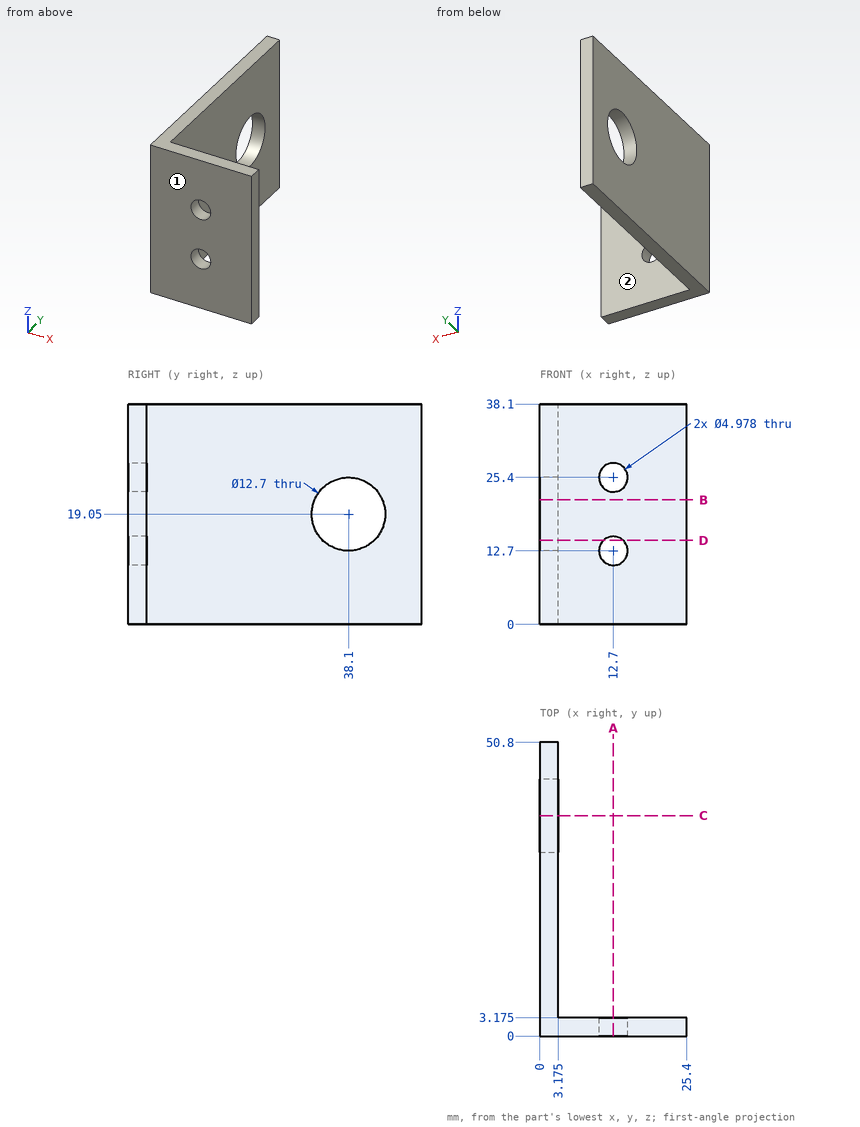
Part print with two shaded views. Sizes in mm from the minimum x, y, z corner. A direction names the side the tool comes from. Round coordinates to 2 decimals unless told otherwise and drop trailing zeros. Order: outer loops, then holes, each group sorted by start corner. A loop starts at its lowest first (then second) coordinate and runs counter-clockwise, first axis right, second up. Notation, with made-up numbers: M -11,-10.75 L 22,-10.75 A26 ccw 22,12.25 Z; hole C -27,-25.75 d3. An arc over 180 degrees is marked long. Answer in a Markdown table with one row per item. Add a question column.
Q1. 3-axis set-ups, long thin cutter, end or side, ignore diameter. For the marked faces 1 and 2: which of +Z, -Z, +X, -X, +Y, -Y reach the whole face in a straight line?
Q2. Cut at C-C on y = 38.1. Give the cut face in (x, z) (1 decimal).
Q3. Wall check: L1, parallel to Z at x = 12.7, y = 1; L2, parallel to Z at x = 1.85, y = 38.1; L3, parallel to X at y = 24, z = 13 (1 decimal). Give the ranges that are in metal, low to high. Write a range as from..to.
Q4. Cut at B-B on z = 21.5. Give the cut face in (x, y) (1 decimal).
Q5. Pin check, flat tips, straight feed: pin 1 (1.5 mm diameter, centred on y = 17.5, z = 11.5, fed in from +X) (3 decimals); pin 2 (2 mm diameter, centred on x = 15.5, z = 17, fed in from +Y) (3 decimals); pin 3 (1 mm diameter, centred on x = 12.5, z = 26, fed in from -Y). Stop position of each tip, or through.
Q6. Cut at D-D on z = 14.5. Give the cut face in (x, y) (1 decimal), and give its area (3 significant figures).
Q7. Cut at A-A on x = 12.7. Give the cut face in (y, z) (1 decimal).
Established:
| question | item | result |
|---|---|---|
| 1 | face 1 | +Z, -Z, +X, -X, -Y |
| 1 | face 2 | +Z, -Z, +X, +Y |
| 2 | outline | M 0,0 L 3.2,0 L 3.2,12.7 L 0,12.7 Z; M 0,25.4 L 3.2,25.4 L 3.2,38.1 L 0,38.1 Z |
| 3 | L1 | z = 0..10.21, 15.19..22.91, 27.89..38.1 |
| 3 | L2 | z = 0..12.7, 25.4..38.1 |
| 3 | L3 | x = 0..3.2 |
| 4 | outline | M 0,0 L 25.4,0 L 25.4,3.2 L 3.2,3.2 L 3.2,32.2 L 0,32.2 Z; M 0,44 L 3.2,44 L 3.2,50.8 L 0,50.8 Z |
| 5 | pin 1 | stops at x = 3.175 |
| 5 | pin 2 | stops at y = 3.175 |
| 5 | pin 3 | passes through |
| 6 | outline | M 0,0 L 11,0 L 11,3.2 L 3.2,3.2 L 3.2,33.7 L 0,33.7 Z; M 0,42.5 L 3.2,42.5 L 3.2,50.8 L 0,50.8 Z; M 14.4,0 L 25.4,0 L 25.4,3.2 L 14.4,3.2 Z |
| 6 | area | 193 mm2 |
| 7 | outline | M 0,0 L 3.2,0 L 3.2,10.2 L 0,10.2 Z; M 0,15.2 L 3.2,15.2 L 3.2,22.9 L 0,22.9 Z; M 0,27.9 L 3.2,27.9 L 3.2,38.1 L 0,38.1 Z |
